For this review, take the finished solid that the model builds, in its own axes (mm). Face numbers are marked on the shaded views. Give positions to 0.01 mm unless a question says otherwise; leave off trailing zeros. Write each loop counter-clockwise with the first axis right and the second up, starting at its lowest first coordinate (ties: lowest second). Pieces come first, ordered by that corner, then holes.
Q1. Mouldability with a two-part tool opening along X and no side actions: class the marked faces 1, 2 and 3 as released by +X, released by -X, zero draft, split by the parting line, or undercut.
Q2. We need section B-B (y = -16.5). Write out the cut boundary in (x, z), then the cut area to 3 significant figures.
Q3. We need section A-A (x = 0). Write out the cut boundary in (y, z), then the cut area to 3 significant figures.
Q4. Insertion check: P1, Ø24, axis at x = 0, y = -10.35, coming from the -Z side. The pin has a flat end and moves straight along its axis. Give the tip position at first contact, or say it passes through.
Q5. We need section C-C (z = 0). Write out the cut boundary in (x, y), then the cut area to 3 significant figures.
Q6. For line 1 (Y direction, x = 0, z = -0.25); line 2 (Y direction, x = -4.5, z = 2); line 3 (X direction, y = -14, z = -2.75), list the stretches that pass through material, from the lowest coordinate up.
```python
from build123d import *

# Parameters (mm, degrees)
SKETCH1_W               = 50.8
SKETCH1_H               = 53.975
BOSS_EXTRUDE1_DEPTH     = 6.35
CUT_EXTRUDE1_DEPTH      = 40.176206507
CUT_EXTRUDE1_DEPTH_BACK = 40.176206507
SKETCH2_R               = 10.499999971
FILLET1_R               = 6.35


with BuildPart() as part:
    # Sketch1 → Boss-Extrude1 (new, symmetric)
    with BuildSketch(Plane.XY):
        Rectangle(SKETCH1_W, SKETCH1_H)
    extrude(amount=BOSS_EXTRUDE1_DEPTH, both=True)

    # Sketch2 → Cut-Extrude1 (cut, two sides: drawn at the far end of the back side and taken through both)
    with BuildSketch(Plane.XY.offset(6.35).offset(-CUT_EXTRUDE1_DEPTH_BACK)):
        with Locations((0, -10.3505)):
            Circle(SKETCH2_R)
    extrude(amount=CUT_EXTRUDE1_DEPTH + CUT_EXTRUDE1_DEPTH_BACK, mode=Mode.SUBTRACT)

    # Fillet1
    fillet1_edges = [part.edges().sort_by_distance(p)[0] for p in [
        (25.4, -26.9875, 0),
        (-25.4, -26.9875, 0),
    ]]
    fillet(fillet1_edges, radius=FILLET1_R)


solid = part.part
```
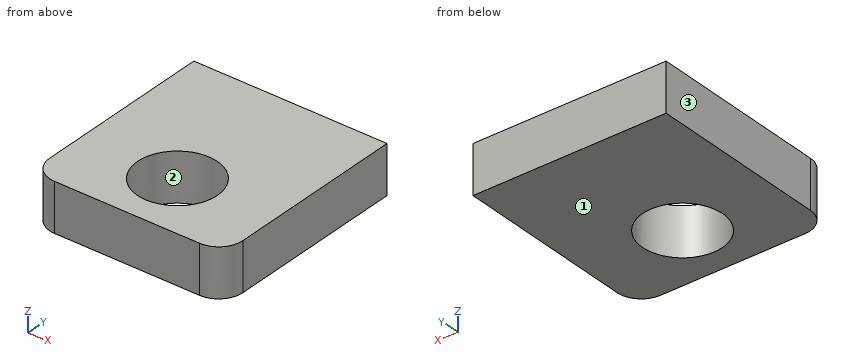
Computed:
1. face 1: zero draft
1. face 2: undercut
1. face 3: released by -X
2. outline: (-25.4, -6.35) - (-8.51, -6.35) - (-8.51, 6.35) - (-25.4, 6.35) - close; (8.51, -6.35) - (25.4, -6.35) - (25.4, 6.35) - (8.51, 6.35) - close
2. area: 429 mm2
3. outline: (-26.99, -6.35) - (-20.85, -6.35) - (-20.85, 6.35) - (-26.99, 6.35) - close; (0.15, -6.35) - (26.99, -6.35) - (26.99, 6.35) - (0.15, 6.35) - close
3. area: 419 mm2
4. P1: stops at z = -6.35
5. outline: (-25.4, -20.64) arc R6.35 ccw to (-19.05, -26.99) - (19.05, -26.99) arc R6.35 ccw to (25.4, -20.64) - (25.4, 26.99) - (-25.4, 26.99) - close; hole circle Ø21 at (0, -10.35)
5. area: 2,380 mm2
6. line 1: y = -26.99 to -20.85, 0.15 to 26.99
6. line 2: y = -26.99 to -19.84, -0.86 to 26.99
6. line 3: x = -25.4 to -9.85, 9.85 to 25.4
